Design review of the part built by this model. Coordinates are the model's own, in mm. A direction names the side the tool comes from. Round coordinates to 2 decimals unless told otherwise and drop trailing zeros. Order: outer loops, then holes, each group sorted by start corner. A loop starts at its lowest first (then second) coordinate and runs counter-clockwise, first axis right, second up. Notation, with made-up numbers: (31, 24) - (40, 24) arc R22 cw to (40, 57) - close; hole circle Ø2 at (6.5, 85). An arc over 180 degrees is marked (long way). Use CSV: the item, a comma, the result in double quotes.
from build123d import *

# Parameters (mm, degrees)
SKETCH2_R           = 10
BOSS_EXTRUDE2_DEPTH = 10
BOSS_EXTRUDE4_DEPTH = 50


with BuildPart() as part:
    # Sketch2 → Boss-Extrude2 (new body)
    with BuildSketch(Plane(origin=(0, 0, 0), x_dir=(1, 0, 0), z_dir=(0, 1, 0))):
        with BuildLine():
            Line((-100, -50), (100, -50))
            Line((100, -50), (100, 30))
            ThreePointArc((100, 30), (94.142135624, 44.142135624), (80, 50))
            Line((80, 50), (-80, 50))
            ThreePointArc((-80, 50), (-94.142135624, 44.142135624), (-100, 30))
            Line((-100, 30), (-100, -50))
        make_face()
        with Locations(Location((58.793969849, 0, 0), (0, 0, 270))):
            Circle(SKETCH2_R, mode=Mode.SUBTRACT)
        with Locations(Location((-60.804020101, 0, 0), (0, 0, 270))):
            Circle(SKETCH2_R, mode=Mode.SUBTRACT)
        with Locations(Location((0, 29.899497487, 0), (0, 0, 270))):
            Circle(SKETCH2_R, mode=Mode.SUBTRACT)
    extrude(amount=BOSS_EXTRUDE2_DEPTH)

    # Sketch3 → Boss-Extrude4 (add)
    with BuildSketch(Plane.XY.offset(50)):
        with BuildLine():
            Line((100, 10), (102.633258285, 10))
            ThreePointArc((102.633258285, 10), (139.989628378, -0.558774103), (102.0351621, -8.710129001))
            Line((102.0351621, -8.710129001), (115.232280048, -8.710129001))
            ThreePointArc((115.232280048, -8.710129001), (128.572143936, 5.229557302), (110.000160919, 0))
            Line((110.000160919, 0), (100, 0))
            Line((100, 0), (-100, 0))
            Line((-100, 0), (-100, 10))
            Line((-100, 10), (100, 10))
        make_face()
    extrude(amount=BOSS_EXTRUDE4_DEPTH)


solid = part.part
1) We need section C-C (y = 7). Give the boundary of the cut face in (x, z).
Data:
outline,"(-100, -30) arc R20 ccw to (-80, -50) - (80, -50) arc R20 ccw to (100, -30) - (100, 50) - (112.78, 50) - (112.78, 100) - (-100, 100) - close; (127.22, 50) - (138.76, 50) - (138.76, 100) - (127.22, 100) - close; hole circle Ø20 at (-60.8, 0); hole circle Ø20 at (0, -29.9); hole circle Ø20 at (58.79, 0)"
2) For faces 1 (the face through (-100, 5, 34)), 2 (the face through (0, 10, 24)), 3 (the face through (100, 5, 11)), list the 3-axis set-ups (+Z, -Z, +X, -X, +Y, -Y) from which the entire face can be reached by the end or side of a thin tool; tool diameter is ignored.
Data:
face 1,"+Z, -Z, -X, +Y, -Y"
face 2,"+Z, -Z, -X, +Y"
face 3,"-Z, +X, +Y, -Y"
3) We need section A-A (z = 0). Give the boundary of the cut face in (x, y), then the cut area to 3 significant figures.
Data:
outline,"(-100, 0) - (-70.8, 0) - (-70.8, 10) - (-100, 10) - close; (-50.8, 0) - (48.79, 0) - (48.79, 10) - (-50.8, 10) - close; (68.79, 0) - (100, 0) - (100, 10) - (68.79, 10) - close"
area,"1,600 mm2"
4) To check wall thickness, follow L1, parallel to X at y = 4.75, z = 0; L2, parallel to X at y = 1, z = 31.5; L3, parallel to Y at x = -71, z = 16.5. State the ranges of each line that lie inside material, in increasing order. Write a range as from..to.
Data:
L1,"x = -100..-70.8, -50.8..48.79, 68.79..100"
L2,"x = -100..100"
L3,"y = 0..10"
5) We need section B-B (x = 0). Give the boundary of the cut face in (y, z), then the cut area to 3 significant figures.
Data:
outline,"(0, -50) - (10, -50) - (10, -39.9) - (0, -39.9) - close; (0, -19.9) - (10, -19.9) - (10, 100) - (0, 100) - close"
area,"1,300 mm2"
6) We need section D-D (z = 70.5). Give the boundary of the cut face in (x, y).
Data:
outline,"(-100, 0) - (110, 0) arc R10 cw (long way) to (115.23, -8.71) - (102.04, -8.71) arc R20 ccw (long way) to (102.63, 10) - (-100, 10) - close"
7) Insertion check: pin 1 Ø2 at (y, z) = (6, 35.5) entering from +X; pin 2 Ø6 at (x, z) = (-41.5, 6) entering from +Y; pin 3 Ø6.5 at (x, z) = (109.5, 64) entering from +Y. Each pin has a flat end and moves straight along its axis. Give the tip position at first contact, or say it passes through.
Data:
pin 1,"stops at x = 100"
pin 2,"stops at y = 10"
pin 3,"stops at y = 18.72"
8) The part is to be moulded in two halves that separate along Z. For faces 4 (the face through (129, 5, 50)), 5 (the face through (3, 4.93, -20.36)), 6 (the face through (-50.89, 4.93, -1.3)), 7 (the face through (109, -8.71, 75)), say which applies: +Z half, -Z half, draft (parallel to the pull), parting line (faces both ways), or undercut.
Data:
face 4,"-Z half"
face 5,"undercut"
face 6,"undercut"
face 7,"draft"
